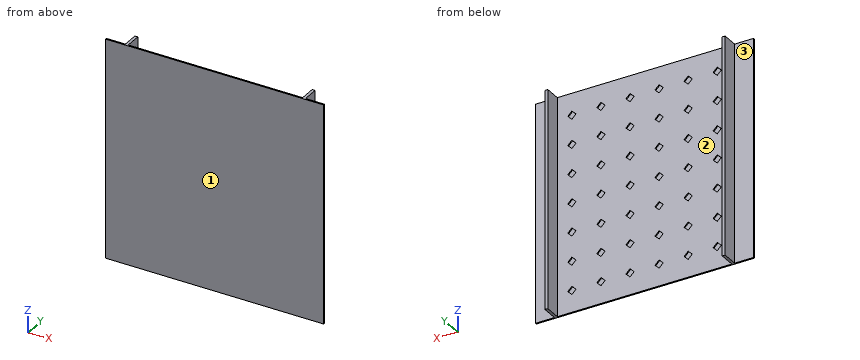
from build123d import *

# Parameters (mm, degrees)
SKETCH2_W           = 1500
SKETCH2_H           = 1500
BOSS_EXTRUDE1_DEPTH = 10
SKETCH3_W           = 20
SKETCH3_H           = 1500
BOSS_EXTRUDE2_DEPTH = 110
CUT_EXTRUDE1_DEPTH  = 8


with BuildPart() as part:
    # Sketch2 → Boss-Extrude1 (new body)
    with BuildSketch(Plane(origin=(0, 0, 0), x_dir=(1, 0, 0), z_dir=(0, 1, 0))):
        Rectangle(SKETCH2_W, SKETCH2_H)
    extrude(amount=BOSS_EXTRUDE1_DEPTH)

    # Sketch3 → Boss-Extrude2 (add)
    with BuildSketch(Plane(origin=(0, 10, 0), x_dir=(1, 0, 0), z_dir=(0, 1, 0))):
        with Locations((-610, 0)):
            Rectangle(SKETCH3_W, SKETCH3_H)
        with Locations((610, 0)):
            Rectangle(SKETCH3_W, SKETCH3_H)
    extrude(amount=BOSS_EXTRUDE2_DEPTH)

    # Sketch4 → Cut-Extrude1 (cut)
    with BuildSketch(Plane(origin=(0, 10, 0), x_dir=(1, 0, 0), z_dir=(0, 1, 0))):
        Polygon((-500, 628.284271247), (-471.715728753, 600), (-500, 571.715728753), (-528.284271247, 600), align=None)
        Polygon((-300, 628.284271247), (-271.715728753, 600), (-300, 571.715728753), (-328.284271247, 600), align=None)
        Polygon((-100, 628.284271247), (-71.715728753, 600), (-100, 571.715728753), (-128.284271247, 600), align=None)
        Polygon((100, 628.284271247), (128.284271247, 600), (100, 571.715728753), (71.715728753, 600), align=None)
        Polygon((300, 628.284271247), (328.284271247, 600), (300, 571.715728753), (271.715728753, 600), align=None)
        Polygon((500, 628.284271247), (528.284271247, 600), (500, 571.715728753), (471.715728753, 600), align=None)
        Polygon((-300, 428.284271247), (-271.715728753, 400), (-300, 371.715728753), (-328.284271247, 400), align=None)
        Polygon((-100, 428.284271247), (-71.715728753, 400), (-100, 371.715728753), (-128.284271247, 400), align=None)
        Polygon((100, 428.284271247), (128.284271247, 400), (100, 371.715728753), (71.715728753, 400), align=None)
        Polygon((300, 428.284271247), (328.284271247, 400), (300, 371.715728753), (271.715728753, 400), align=None)
        Polygon((500, 428.284271247), (528.284271247, 400), (500, 371.715728753), (471.715728753, 400), align=None)
        Polygon((-300, 228.284271247), (-271.715728753, 200), (-300, 171.715728753), (-328.284271247, 200), align=None)
        Polygon((-100, 228.284271247), (-71.715728753, 200), (-100, 171.715728753), (-128.284271247, 200), align=None)
        Polygon((100, 228.284271247), (128.284271247, 200), (100, 171.715728753), (71.715728753, 200), align=None)
        Polygon((300, 228.284271247), (328.284271247, 200), (300, 171.715728753), (271.715728753, 200), align=None)
        Polygon((500, 228.284271247), (528.284271247, 200), (500, 171.715728753), (471.715728753, 200), align=None)
        Polygon((-300, 28.284271247), (-271.715728753, 0), (-300, -28.284271247), (-328.284271247, 0), align=None)
        Polygon((-100, 28.284271247), (-71.715728753, 0), (-100, -28.284271247), (-128.284271247, 0), align=None)
        Polygon((100, 28.284271247), (128.284271247, 0), (100, -28.284271247), (71.715728753, 0), align=None)
        Polygon((300, 28.284271247), (328.284271247, 0), (300, -28.284271247), (271.715728753, 0), align=None)
        Polygon((500, 28.284271247), (528.284271247, 0), (500, -28.284271247), (471.715728753, 0), align=None)
        Polygon((-300, -171.715728753), (-271.715728753, -200), (-300, -228.284271247), (-328.284271247, -200), align=None)
        Polygon((-100, -171.715728753), (-71.715728753, -200), (-100, -228.284271247), (-128.284271247, -200), align=None)
        Polygon((100, -171.715728753), (128.284271247, -200), (100, -228.284271247), (71.715728753, -200), align=None)
        Polygon((300, -171.715728753), (328.284271247, -200), (300, -228.284271247), (271.715728753, -200), align=None)
        Polygon((500, -171.715728753), (528.284271247, -200), (500, -228.284271247), (471.715728753, -200), align=None)
        Polygon((-300, -371.715728753), (-271.715728753, -400), (-300, -428.284271247), (-328.284271247, -400), align=None)
        Polygon((-100, -371.715728753), (-71.715728753, -400), (-100, -428.284271247), (-128.284271247, -400), align=None)
        Polygon((100, -371.715728753), (128.284271247, -400), (100, -428.284271247), (71.715728753, -400), align=None)
        Polygon((300, -371.715728753), (328.284271247, -400), (300, -428.284271247), (271.715728753, -400), align=None)
        Polygon((500, -371.715728753), (528.284271247, -400), (500, -428.284271247), (471.715728753, -400), align=None)
        Polygon((-500, 428.284271247), (-471.715728753, 400), (-500, 371.715728753), (-528.284271247, 400), align=None)
        Polygon((-500, 228.284271247), (-471.715728753, 200), (-500, 171.715728753), (-528.284271247, 200), align=None)
        Polygon((-500, 28.284271247), (-471.715728753, 0), (-500, -28.284271247), (-528.284271247, 0), align=None)
        Polygon((-500, -171.715728753), (-471.715728753, -200), (-500, -228.284271247), (-528.284271247, -200), align=None)
        Polygon((-500, -371.715728753), (-471.715728753, -400), (-500, -428.284271247), (-528.284271247, -400), align=None)
        Polygon((-500, -571.715728753), (-471.715728753, -600), (-500, -628.284271247), (-528.284271247, -600), align=None)
        Polygon((-300, -571.715728753), (-271.715728753, -600), (-300, -628.284271247), (-328.284271247, -600), align=None)
        Polygon((-100, -571.715728753), (-71.715728753, -600), (-100, -628.284271247), (-128.284271247, -600), align=None)
        Polygon((100, -571.715728753), (128.284271247, -600), (100, -628.284271247), (71.715728753, -600), align=None)
        Polygon((300, -571.715728753), (328.284271247, -600), (300, -628.284271247), (271.715728753, -600), align=None)
        Polygon((500, -571.715728753), (528.284271247, -600), (500, -628.284271247), (471.715728753, -600), align=None)
    extrude(amount=-CUT_EXTRUDE1_DEPTH, mode=Mode.SUBTRACT)


solid = part.part
Design review of the part built by this model. Coordinates are the model's own, in mm. Face numbers are marked on the shaded views. A direction names the side the tool comes from. Give positions to 0.01 mm unless a question says otherwise; leave off trailing zeros. Order: outer loops, then holes, each group sorted by start corner. A loop starts at its lowest first (then second) coordinate and runs counter-clockwise, first axis right, second up. Notation, with made-up numbers: (49, 3.25) - (99, 3.25) arc R27 cw to (99, 29.25) - close; hole circle Ø1 at (82, 3.25). An arc over 180 degrees is marked (long way). Write item = value, one per line. Start each with the question number.
Q1. We need section B-B on z = 654.5. State the section outline as (x, y) points.
Q2. Tool access review of the marked faces 1, 2 and 3: name each direction out of +Z, -Z, +X, -X, +Y, -Y from which nothing blocks a thin tool from reaching the whole face with its end or side.
Q3. We need section A-A on y = 55. State the section outline as (x, z) points.
Q4. Clearance check with flat-ended pins moving along their axes: pin 1 Ø6 at (y, z) = (105.5, 34) entering from +X; pin 2 Ø5 at (y, z) = (67.5, -96.5) entering from -X; pin 3 Ø17 at (x, z) = (-105.5, -607) entering from +Y. State where each tip first meets the part, or that it passes through.
Q5. We need section C-C on x = -39. State the section outline as (y, z) points.
Q6. To check wall thickness, follow L1, parallel to X at y = 79, z = 468.5; L2, parallel to Y at x = -151.5, z = -7. State the ranges of each line that lie inside material, in increasing order. Write a range as from..to.
Working result:
q1.outline = (-750, 0) - (750, 0) - (750, 10) - (620, 10) - (620, 120) - (600, 120) - (600, 10) - (-600, 10) - (-600, 120) - (-620, 120) - (-620, 10) - (-750, 10) - close
q2.face_1 = +Z, -Z, +X, -X, -Y
q2.face_2 = +Z, -Z, +Y
q2.face_3 = +Z, -Z, -X, +Y
q3.outline = (-620, -750) - (-600, -750) - (-600, 750) - (-620, 750) - close; (600, -750) - (620, -750) - (620, 750) - (600, 750) - close
q4.pin_1 = 620
q4.pin_2 = -620
q4.pin_3 = 2
q5.outline = (0, -750) - (10, -750) - (10, 750) - (0, 750) - close
q6.L1 = -620..-600, 600..620
q6.L2 = 0..10
